Read the model definition and answer for the solid it produces. Units are mm, in the model's axes. Give positions to 0.01 mm unless a question says otherwise; leave off trailing zeros. Order: outer loops, then holes, each group sorted by start corner. A loop starts at its lowest first (then second) coordinate and runs counter-clockwise, first axis right, second up.
```python
from build123d import *

# Parameters (mm, degrees)
F0_R     = 571.5
F1_DEPTH = 12.7
F2_DEPTH = 3.81


# Not quite as in the source:
# - a fillet or chamfer that OpenCascade refuses, or shapes differently, is made with other operations: its cross-section is extruded or revolved along the edge and cut away or added


with BuildPart() as f1:
    # F0 (on Top) → F1 (new body)
    with BuildSketch(Plane.XY):
        Circle(F0_R)
    extrude(amount=F1_DEPTH)

    # F2 (add): a face of the model
    f2_faces = [f1.faces().sort_by_distance(p)[0] for p in [
        (0, 0, 12.7),
    ]]
    extrude(f2_faces, amount=F2_DEPTH)

    # F3: chamfer of 25.4 on 1 edges, made by hand

    # F3_s1 → F3_t2 (revolve, cut)
    with BuildSketch(Plane.XZ):
        Polygon((571.5, -8.89), (546.1, 16.51), (571.5, 16.51), align=None)
    revolve(axis=Axis((0, 0, 16.51), (0, 0, 1)), mode=Mode.SUBTRACT)


solid = f1.part
```
1) The part is cut by section A-A on z = 8. Determine the outline of the cut face in (x, y), and give its area (3 significant figures).
Final values:
outline: circle Ø1109.22 at (0, 0)
area: 966,000 mm2
2) Consider L1, parallel to Y at x = -486.5, z = 2.25; L2, parallel to X at y = -254, z = 1.25; L3, parallel to X at y = -196, z = 9.25. Determine where each line is inside the solid, lowest interval first.
Final values:
L1: y = -278.07 to 278.07
L2: x = -500.61 to 500.61
L3: x = -517.49 to 517.49
3) Given pin 1 (8 mm diameter, centred on x = -442, z = 7.5, fed in from -Y); pin 2 (3 mm diameter, centred on x = -26, z = 9, fed in from -Y); pin 3 (2 mm diameter, centred on y = 231.5, z = 9, fed in from +X), each flat-ended and moving along its own axis, determine where each tip first touches the part or whether it passes through.
Final values:
pin 1: stops at y = -344.19
pin 2: stops at y = -554.5
pin 3: stops at x = 504.08
